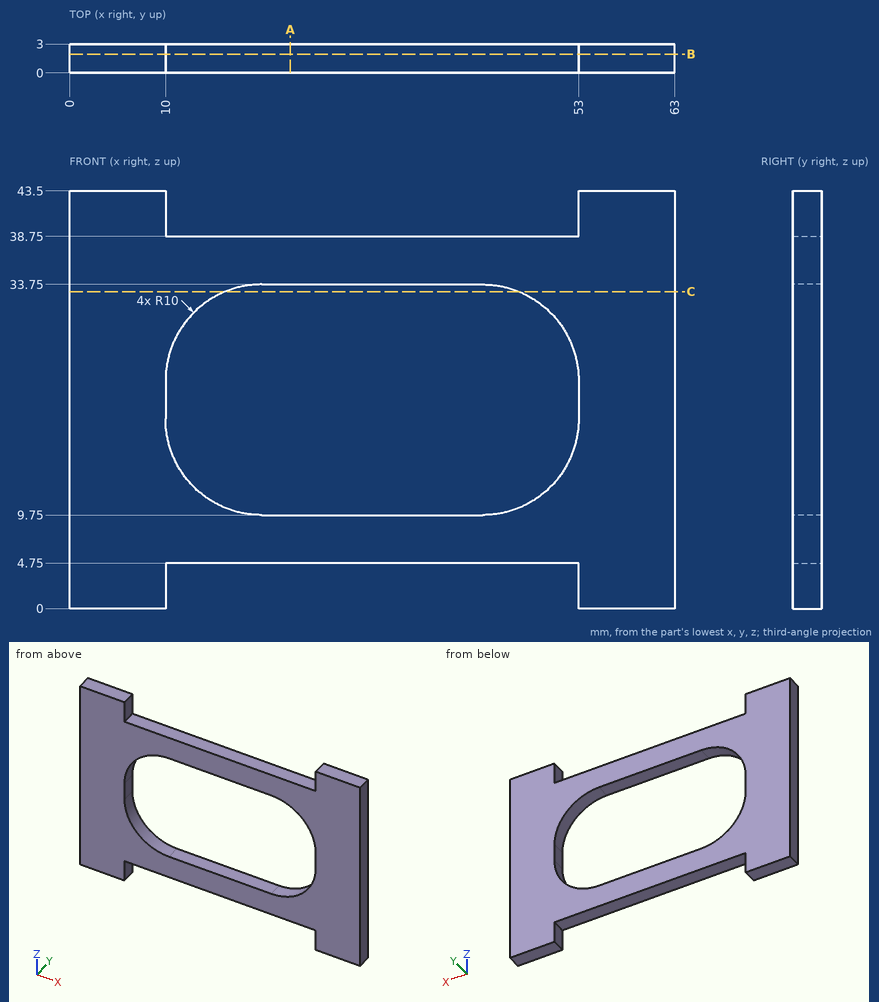
Can you work these out from the drawing? Everything is in mm from the part's minimum corner. Give positions to 0.01 mm unless a question says otherwise; leave off trailing zeros. Order: outer loops, then holes, each group sorted by start corner. A loop starts at its lowest first (then second) coordinate and runs counter-clockwise, first axis right, second up. Notation, with made-up numbers: M 72.25,5 L 94.25,5 A33 ccw 94.25,40 Z; hole C 88.5,38.5 d2. An arc over 180 degrees is marked long. One line per item, written item: value.
Item 1: For pin 1 (0.9 mm diameter, centred on y = 1, z = 1.5, fed in from -X); pin 2 (1.5 mm diameter, centred on x = 28, y = 1, fed in from -Z); pin 3 (0.9 mm diameter, centred on x = 32.5, y = 1.5, fed in from +Z), each with a flat end and sliding along its axis, tell me the tip position at first contact or that it passes through.
Verdict:
pin 1: x = 0
pin 2: z = 4.75
pin 3: z = 38.75
Item 2: If we section it at B-B on y = 1.95: Write out the boundary of the cut face in (x, z), and give its area (3 significant figures).
Verdict:
outline: M 0,0 L 10,0 L 10,4.75 L 53,4.75 L 53,0 L 63,0 L 63,43.5 L 53,43.5 L 53,38.75 L 10,38.75 L 10,43.5 L 0,43.5 Z; hole M 10,19.75 A10 ccw 20,9.75 L 43,9.75 A10 ccw 53,19.75 L 53,23.75 A10 ccw 43,33.75 L 20,33.75 A10 ccw 10,23.75 Z
area: 1,390 mm2
Item 3: If we section it at A-A on x = 23: Write out the boundary of the cut face in (y, z), and give its area (3 significant figures).
Verdict:
outline: M 0,4.75 L 3,4.75 L 3,9.75 L 0,9.75 Z; M 0,33.75 L 3,33.75 L 3,38.75 L 0,38.75 Z
area: 30.0 mm2
Item 4: Please list where these lines run through material, in increasing order: line 1 (Z direction, x = 36, y = 0.6); line 2 (X direction, y = 0.4, z = 41); line 3 (X direction, y = 1.8, z = 16.5).
Verdict:
line 1: 4.75 to 9.75, 33.75 to 38.75
line 2: 0 to 10, 53 to 63
line 3: 0 to 10.54, 52.46 to 63
Item 5: If we section it at C-C on z = 33: Write out the boundary of the cut face in (x, y).
Verdict:
outline: M 0,0 L 16.2,0 L 16.2,3 L 0,3 Z; M 46.8,0 L 63,0 L 63,3 L 46.8,3 Z
